```python
from build123d import *

# Parameters (mm, degrees)
F3_D     = 6.6
F5_D     = 17.4
F5_DEPTH = 12
F5_TIP   = 5.2274873855
F6_D     = 19
F6_DEPTH = 5
F6_TIP   = 5.7081758808
F7_DEPTH = 25
F8_R     = 3


with BuildPart() as f1:
    # F0 (on Right) → F1 (revolve)
    with BuildSketch(Plane.YZ):
        Polygon((-30, 0), (0, 0), (0, 30), (-30, 10), align=None)
    revolve(axis=Axis((0, -15, 0), (0, -1, 0)))

    # F3 (through all)
    with Locations(Plane.XZ.offset(30)):
        with Locations((0, 0)):
            Hole(F3_D / 2)

    # F5
    with Locations(Plane(origin=(0, 0, 0), x_dir=(-1, 0, 0), z_dir=(0, 1, 0))):
        with Locations((0, 0)):
            Hole(F5_D / 2, depth=F5_DEPTH)
            with Locations((0, 0, -(F5_DEPTH + F5_TIP / 2))):  # 118° drill point
                Cone(0, F5_D / 2, F5_TIP, mode=Mode.SUBTRACT)

    # F6
    with Locations(Plane(origin=(0, 0, 0), x_dir=(-1, 0, 0), z_dir=(0, 1, 0))):
        with Locations((0, 0)):
            Hole(F6_D / 2, depth=F6_DEPTH)
            with Locations((0, 0, -(F6_DEPTH + F6_TIP / 2))):  # 118° drill point
                Cone(0, F6_D / 2, F6_TIP, mode=Mode.SUBTRACT)

    # F2 (on face) → F7 (cut)
    with BuildSketch(Plane.XZ.offset(30)):
        with BuildLine():
            ThreePointArc((11.313708499, -4), (8.4852813742, -8.4852813742), (4, -11.313708499))
            Line((4, -11.313708499), (4, -27.313708499))
            ThreePointArc((4, -27.313708499), (19.5197165959, -19.5197165959), (27.313708499, -4))
            Line((27.313708499, -4), (11.313708499, -4))
        make_face()
        with BuildLine():
            Line((11.313708499, 4), (27.313708499, 4))
            ThreePointArc((27.313708499, 4), (19.5197165959, 19.5197165959), (4, 27.313708499))
            Line((4, 27.313708499), (4, 11.313708499))
            ThreePointArc((4, 11.313708499), (8.4852813742, 8.4852813742), (11.313708499, 4))
        make_face()
        with BuildLine():
            Line((-4, 11.313708499), (-4, 27.313708499))
            ThreePointArc((-4, 27.313708499), (-19.5197165959, 19.5197165959), (-27.313708499, 4))
            Line((-27.313708499, 4), (-11.313708499, 4))
            ThreePointArc((-11.313708499, 4), (-8.4852813742, 8.4852813742), (-4, 11.313708499))
        make_face()
        with BuildLine():
            Line((-11.313708499, -4), (-27.313708499, -4))
            ThreePointArc((-27.313708499, -4), (-19.5197165959, -19.5197165959), (-4, -27.313708499))
            Line((-4, -27.313708499), (-4, -11.313708499))
            ThreePointArc((-4, -11.313708499), (-8.4852813742, -8.4852813742), (-11.313708499, -4))
        make_face()
    extrude(amount=-F7_DEPTH, mode=Mode.SUBTRACT)

    # F8
    f8_edges = [f1.edges().sort_by_distance(p)[0] for p in [
        (0, 0, -30),
        (0, -30, -10),
    ]]
    fillet(f8_edges, radius=F8_R)


solid = f1.part
```
Build history of the part. All positions in model axes, mm. A direction names the side the tool comes from. Round coordinates to 2 decimals unless told otherwise and drop trailing zeros. Write each loop counter-clockwise with the first axis right and the second up, starting at its lowest first coordinate (ties: lowest second). Pieces come first, ordered by that corner, then holes. Notation, with made-up numbers: (-16.5, -8) - (-4.5, -8) arc R29 ccw to (-4.5, 14) - close; hole circle Ø10 at (27, 69.5). An arc over 180 degrees is marked (long way). Write each question's results on one line, items separated by ' | '. Start each with the question number.
Item 1: Drop flat-ended pins along their axis: P1, Ø6.5, axis at x = 14.5, z = -13.5, coming from the -Y side; P2, Ø1.5, axis at x = 14, y = -7.5, coming from the -Z side; P3, Ø12, axis at y = -26.5, z = -3.5, coming from the -X side. Give the stop position or say it passes through.
Item 2: Which spindle directions (+Z, -Z, +X, -X, +Y, -Y) get a long thin tool onto all of the face, cutting with end or side? Do faces 1 (the face through (4, -11, 16)), 2 (the face through (-8.54, -16.15, 8.43)), 3 (the face through (8.54, -16.15, -8.43)), 4 (the face through (-4, -11, -16)). Say none if no direction does.
Item 3: Mould opens along Z. For faces 5 (the face through (17, -14, 4)), 6 (the face through (0, 0, -11)), 7 (the face through (4.38, -2.54, -8.43)) say: pulls with the +Z half, pulls with the -Z half, needs draft (parallel to the pull), parting line crosses it, or undercut.
Item 4: Wall check: L1, parallel to X at y = -2.75, z = 0; L2, parallel to X at y = -8.25, z = 24; L3, parallel to Y at x = -10, z = 9. Give the ranges that are in metal, low to high. Write a range as [from, to].
Item 5: Saw through at C-C (y = -18.5). Write the cut outline in (x, z), and give its area (3 significant figures).
Item 6: Saw through at A-A (z = 0). Write the cut outline in (x, y).
Item 7: Saw through at D-D (y = -14.25). Write the cut outline in (x, z), and give its area (3 significant figures).
Item 8: Saw through at B-B (x = 0). Write the cut outline in (y, z).
Results are:
1) P1: stops at y = -5 | P2: stops at z = -4 | P3: stops at x = -16.09
2) face 1: +Z, +X, -Y | face 2: +Z, -X, -Y | face 3: -Z, +X, -Y | face 4: -Z, -X, -Y
3) face 5: pulls with the +Z half | face 6: needs draft | face 7: undercut
4) L1: x = [-27.38, -9.5], [9.5, 27.38] | L2: x = [-4, 4] | L3: y = [-5, 0]
5) outline: (-17.21, -4) - (-11.31, -4) arc R12 ccw to (-4, -11.31) - (-4, -17.21) arc R17.67 ccw to (4, -17.21) - (4, -11.31) arc R12 ccw to (11.31, -4) - (17.21, -4) arc R17.67 ccw to (17.21, 4) - (11.31, 4) arc R12 ccw to (4, 11.31) - (4, 17.21) arc R17.67 ccw to (-4, 17.21) - (-4, 11.31) arc R12 ccw to (-11.31, 4) - (-17.21, 4) arc R17.67 ccw to start; hole circle Ø6.6 at (0, 0) | area: 602 mm²
6) outline: (-26.89, -4.66) - (-10.89, -28.66) arc R3 ccw to (-8.39, -30) - (-3.3, -30) - (-3.3, -15.24) - (-8.7, -12) - (-8.7, -5.48) - (-9.5, -5) - (-9.5, 0) - (-24.39, 0) arc R3 ccw to start; (3.3, -30) - (8.39, -30) arc R3 ccw to (10.89, -28.66) - (26.89, -4.66) arc R3 ccw to (24.39, 0) - (9.5, 0) - (9.5, -5) - (8.7, -5.48) - (8.7, -12) - (3.3, -15.24) - close
7) outline: (-20.11, -4) - (-11.31, -4) arc R12 ccw to (-4, -11.31) - (-4, -20.11) arc R20.5 ccw to (4, -20.11) - (4, -11.31) arc R12 ccw to (11.31, -4) - (20.11, -4) arc R20.5 ccw to (20.11, 4) - (11.31, 4) arc R12 ccw to (4, 11.31) - (4, 20.11) arc R20.5 ccw to (-4, 20.11) - (-4, 11.31) arc R12 ccw to (-11.31, 4) - (-20.11, 4) arc R20.5 ccw to start; hole circle Ø9.91 at (0, 0) | area: 650 mm²
8) outline: (-30, -8.39) arc R3 ccw to (-28.66, -10.89) - (-4.66, -26.89) arc R3 ccw to (0, -24.39) - (0, -9.5) - (-5, -9.5) - (-5.48, -8.7) - (-12, -8.7) - (-15.24, -3.3) - (-30, -3.3) - close; (-30, 3.3) - (-15.24, 3.3) - (-12, 8.7) - (-5.48, 8.7) - (-5, 9.5) - (0, 9.5) - (0, 24.39) arc R3 ccw to (-4.66, 26.89) - (-28.66, 10.89) arc R3 ccw to (-30, 8.39) - close
